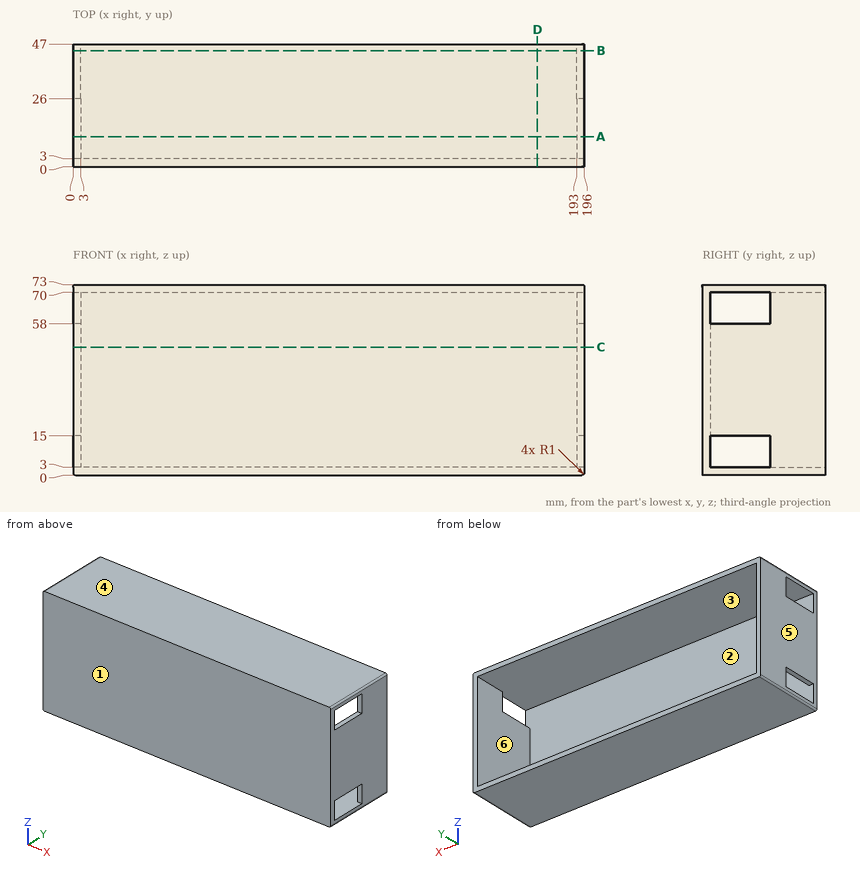
For this review, use the dimensioned drawing (mm, ordinates from the lowest corner) and the shaded views. A direction names the side the tool comes from. Give positions to 0.01 mm unless a question says otherwise; leave off trailing zeros. Loops run counter-clockwise (first coordinate to the right, second up) from the corner with the lowest first, then second, coordinate; pieces in that order, holes last. Notation, with made-up numbers: (-6.5, -39.75) -> (51.5, -39.75) arc R5 cw to (51.5, -32.75) -> close; hole circle Ø7 at (-38.75, 13). An arc over 180 degrees is marked (long way). Use CSV: the item, a comma, the result in double quotes.
1. The part is to be moulded in two halves that separate along Z. For the marked faces 1, 2, 3 and 4, say which applies: +Z half, -Z half, draft (parallel to the pull), parting line (faces both ways), or undercut.
Result:
face 1,"draft"
face 2,"undercut"
face 3,"undercut"
face 4,"+Z half"
2. Machinability: for the marked faces 5 and 6, which of the approach directions +Z, -Z, +X, -X, +Y, -Y give a long, thin tool a straight path to every point of the face, cutting with its end or side? Answer none if there is none.
Result:
face 5,"+Z, -Z, -X, +Y, -Y"
face 6,"+Y"
3. Consider section C-C, the plane z = 49. Write out the cut boundary in (x, y), then the cut area to 3 significant figures.
Result:
outline,"(0, 0) -> (196, 0) -> (196, 47) -> (193, 47) -> (193, 3) -> (3, 3) -> (3, 47) -> (0, 47) -> close"
area,"852 mm²"
4. For P1, Ø1.5, axis at x = 2, y = 12, coming from the -Z side; P2, Ø3, axis at x = 111, z = 60.5, coming from the +Y side, all flat-tipped, find the tip position at first contact; note any pin that passes through.
Result:
P1,"stops at z = 0"
P2,"stops at y = 3"
5. To check wall thickness, follow probe 1 along X at (y, z) = (33, 69); probe 2 along Z at (x, y) = (54.5, 33); probe 3 along Y at (x, z) = (46.5, 22). State the ranges of each line that lie inside material, in increasing order. Write a range as from..to.
Result:
probe 1,"x = 0..3, 193..196"
probe 2,"z = 0..3, 70..73"
probe 3,"y = 0..3"
6. Consider section A-A, the plane y = 11.5. Write out the cut boundary in (x, z), then the cut area to 3 significant figures.
Result:
outline,"(0, 1) arc R1 ccw to (1, 0) -> (195, 0) arc R1 ccw to (196, 1) -> (196, 3) -> (0, 3) -> close; (0, 15) -> (3, 15) -> (3, 58) -> (0, 58) -> close; (0, 70) -> (196, 70) -> (196, 72) arc R1 ccw to (195, 73) -> (1, 73) arc R1 ccw to (0, 72) -> close; (193, 15) -> (196, 15) -> (196, 58) -> (193, 58) -> close"
area,"1,430 mm²"
7. Consider section D-D, the plane x = 178. Write out the cut boundary in (y, z), then the cut area to 3 significant figures.
Result:
outline,"(0, 0) -> (47, 0) -> (47, 3) -> (3, 3) -> (3, 70) -> (47, 70) -> (47, 73) -> (0, 73) -> close"
area,"483 mm²"
8. Consider section B-B, the plane y = 44.5. Write out the cut boundary in (x, z).
Result:
outline,"(0, 1) arc R1 ccw to (1, 0) -> (195, 0) arc R1 ccw to (196, 1) -> (196, 72) arc R1 ccw to (195, 73) -> (1, 73) arc R1 ccw to (0, 72) -> close; hole (3, 3) -> (193, 3) -> (193, 70) -> (3, 70) -> close"
